```python
from build123d import *

# Parameters (mm, degrees)
F1_DEPTH = 25.4
F2_DEPTH = 25.4
F3_DEPTH = 25.4


with BuildPart() as f1:
    # F0 (on Front) → F1 (new body)
    with BuildSketch(Plane.XZ):
        with BuildLine():
            ThreePointArc((-4.7244, 0), (-18.194785, -5.579616), (-23.7744, -19.05))
            Line((-23.7744, -19.05), (-23.7744, -38.1))
            Line((-23.7744, -38.1), (-17.4244, -38.1))
            Line((-17.4244, -38.1), (-17.4244, -24.509516))
            ThreePointArc((-17.4244, -24.509516), (-18.201369, -19.999674), (-17.4244, -15.489832))
            Line((-17.4244, -15.489832), (-17.4244, -6.35))
            Line((-17.4244, -6.35), (7.9756, -6.35))
            Line((7.9756, -6.35), (7.9756, -15.489832))
            ThreePointArc((7.9756, -15.489832), (8.752568, -19.999674), (7.9756, -24.509516))
            Line((7.9756, -24.509516), (7.9756, -38.1))
            Line((7.9756, -38.1), (14.3256, -38.1))
            Line((14.3256, -38.1), (14.3256, -19.05))
            ThreePointArc((14.3256, -19.05), (8.745984, -5.579616), (-4.7244, 0))
        make_face()
    extrude(amount=F1_DEPTH)

    # F0 (on Front) → F2 (join)
    with BuildSketch(Plane.XZ):
        with BuildLine():
            ThreePointArc((-4.7244, 0), (-18.194785, -5.579616), (-23.7744, -19.05))
            Line((-23.7744, -19.05), (-23.7744, -38.1))
            Line((-23.7744, -38.1), (-17.4244, -38.1))
            Line((-17.4244, -38.1), (-17.4244, -24.509516))
            ThreePointArc((-17.4244, -24.509516), (-18.201369, -19.999674), (-17.4244, -15.489832))
            Line((-17.4244, -15.489832), (-17.4244, -6.35))
            Line((-17.4244, -6.35), (7.9756, -6.35))
            Line((7.9756, -6.35), (7.9756, -15.489832))
            ThreePointArc((7.9756, -15.489832), (8.752568, -19.999674), (7.9756, -24.509516))
            Line((7.9756, -24.509516), (7.9756, -38.1))
            Line((7.9756, -38.1), (14.3256, -38.1))
            Line((14.3256, -38.1), (14.3256, -19.05))
            ThreePointArc((14.3256, -19.05), (8.745984, -5.579616), (-4.7244, 0))
        make_face()
        with BuildLine():
            ThreePointArc((-17.4244, -15.489832), (-18.201369, -19.999674), (-17.4244, -24.509516))
            Line((-17.4244, -24.509516), (-17.4244, -15.489832))
        make_face()
        with BuildLine():
            Line((-17.4244, -6.35), (-17.4244, -15.489832))
            ThreePointArc((-17.4244, -15.489832), (-4.7244, -6.522705), (7.9756, -15.489832))
            Line((7.9756, -15.489832), (7.9756, -6.35))
            Line((7.9756, -6.35), (-17.4244, -6.35))
        make_face()
        with BuildLine():
            ThreePointArc((7.9756, -24.509516), (8.752568, -19.999674), (7.9756, -15.489832))
            Line((7.9756, -15.489832), (7.9756, -24.509516))
        make_face()
    extrude(amount=F2_DEPTH)

    # F0 (on Front) → F3 (join)
    with BuildSketch(Plane.XZ):
        with BuildLine():
            ThreePointArc((-4.7244, 0), (-18.194785, -5.579616), (-23.7744, -19.05))
            Line((-23.7744, -19.05), (-23.7744, -38.1))
            Line((-23.7744, -38.1), (-17.4244, -38.1))
            Line((-17.4244, -38.1), (-17.4244, -24.509516))
            ThreePointArc((-17.4244, -24.509516), (-18.201369, -19.999674), (-17.4244, -15.489832))
            Line((-17.4244, -15.489832), (-17.4244, -6.35))
            Line((-17.4244, -6.35), (7.9756, -6.35))
            Line((7.9756, -6.35), (7.9756, -15.489832))
            ThreePointArc((7.9756, -15.489832), (8.752568, -19.999674), (7.9756, -24.509516))
            Line((7.9756, -24.509516), (7.9756, -38.1))
            Line((7.9756, -38.1), (14.3256, -38.1))
            Line((14.3256, -38.1), (14.3256, -19.05))
            ThreePointArc((14.3256, -19.05), (8.745984, -5.579616), (-4.7244, 0))
        make_face()
        with BuildLine():
            ThreePointArc((-17.4244, -15.489832), (-18.201369, -19.999674), (-17.4244, -24.509516))
            Line((-17.4244, -24.509516), (-17.4244, -15.489832))
        make_face()
        with BuildLine():
            Line((-17.4244, -6.35), (-17.4244, -15.489832))
            ThreePointArc((-17.4244, -15.489832), (-4.7244, -6.522705), (7.9756, -15.489832))
            Line((7.9756, -15.489832), (7.9756, -6.35))
            Line((7.9756, -6.35), (-17.4244, -6.35))
        make_face()
        with BuildLine():
            ThreePointArc((7.9756, -24.509516), (8.752568, -19.999674), (7.9756, -15.489832))
            Line((7.9756, -15.489832), (7.9756, -24.509516))
        make_face()
    extrude(amount=F3_DEPTH)


solid = f1.part
```
Work out the finished part from the listing and answer in its coordinate system (mm). Round coordinates to 2 decimals unless told otherwise and drop trailing zeros. Write each loop counter-clockwise with the first axis right and the second up, starting at its lowest first coordinate (ties: lowest second). Pieces come first, ordered by that corner, then holes. Notation, with made-up numbers: (89, 60.5) -> (121, 60.5) arc R13 cw to (121, 72.5) -> close; hole circle Ø9 at (-34, 81.5). An arc over 180 degrees is marked (long way). Write each question's results on one line, items separated by ' | '.
1) For a pull along X with two mould halves and no side action, classify faces 1 (the flat face through (7.976, -13, -27)), 2 (the flat face through (-17.424, -13, -27)), 3 (the flat face through (11, -13, -38.1)), 4 (the flat face through (14.326, -13, -29)) as +X half, -X half, draft (parallel to the pull), parting line (faces both ways), or undercut.
Findings:
face 1: undercut | face 2: undercut | face 3: draft | face 4: +X half
2) The part is cut by section D-D (x = -9.5). Write down the section's boundary in (y, z).
Findings:
outline: (-25.4, -7.4) -> (0, -7.4) -> (0, -0.61) -> (-25.4, -0.61) -> close
3) Consider line 1 along X through (y, z) = (-2.5, -31); line 2 along X through (y, z) = (-7, -13); line 3 along Z through (x, y) = (-9.5, -7). Determine where each line is inside the solid, lowest interval first. Write a range as [from, to].
Findings:
line 1: x = [-23.77, -17.42], [7.98, 14.33] | line 2: x = [-22.79, -16.24], [6.79, 13.34] | line 3: z = [-7.4, -0.61]
4) Flat-ended cylindrical pins translate along their axes: pin 1 (2 mm diameter, centred on y = -3, z = -4.5, fed in from -X); pin 2 (10 mm diameter, centred on y = -5.5, z = -13, fed in from -X); pin 3 (2 mm diameter, centred on x = -16, y = -8, fed in from -Z); pin 4 (5 mm diameter, centred on x = 8, z = -13.5, fed in from +Y). Find the tip coordinate at first contact, or state that the pin passes through.
Findings:
pin 1: stops at x = -18.11 | pin 2: stops at x = -23.75 | pin 3: stops at z = -14.44 | pin 4: stops at y = 0
5) The part is cut by section C-C (z = -13.5). Write down the section's boundary in (x, y), and give its area (3 significant figures).
Findings:
outline: (-22.95, -25.4) -> (-16.53, -25.4) -> (-16.53, 0) -> (-22.95, 0) -> close; (7.08, -25.4) -> (13.5, -25.4) -> (13.5, 0) -> (7.08, 0) -> close | area: 326 mm²
6) The part is cut by section B-B (y = -7). Write down the section's boundary in (x, z).
Findings:
outline: (-23.77, -38.1) -> (-17.42, -38.1) -> (-17.42, -15.49) arc R13.48 cw to (7.98, -15.49) -> (7.98, -38.1) -> (14.33, -38.1) -> (14.33, -19.05) arc R19.05 ccw to (-4.72, 0) arc R19.05 ccw to (-23.77, -19.05) -> close
7) The part is cut by section A-A (z = -27). Write down the section's boundary in (x, y), and give its area (3 significant figures).
Findings:
outline: (-23.77, -25.4) -> (-17.42, -25.4) -> (-17.42, 0) -> (-23.77, 0) -> close; (7.98, -25.4) -> (14.33, -25.4) -> (14.33, 0) -> (7.98, 0) -> close | area: 323 mm²
